from build123d import *

# Parameters (mm, degrees)
SKETCH2_W                       = 110
SKETCH2_H                       = 110
BOSS_EXTRUDE1_DEPTH             = 5.5
BOSS_EXTRUDE2_DEPTH             = 14
CUT_EXTRUDE5_REACH              = 110.823
SKETCH9_R                       = 1.3
CUT_EXTRUDE6_DEPTH              = 7.5
CUT_EXTRUDE9_REACH              = 109.547
SKETCH11_R                      = 9
BOSS_EXTRUDE7_DEPTH             = 9
BOSS_EXTRUDE7_DIRECTION_2_REACH = 119.904
BOSS_EXTRUDE10_DEPTH            = 9
CUT_EXTRUDE10_DEPTH             = 3.5
F_4_0_4_DIAMETER_HOLE3_D        = 4
FILLET1_R                       = 27.5
FILLET2_R                       = 40


with BuildPart() as part:
    # Sketch2 → Boss-Extrude1 (new body)
    with BuildSketch(Plane(origin=(0, 0, 0), x_dir=(1, 0, 0), z_dir=(0, 1, 0))):
        with Locations((-8.65, 8.65)):
            Rectangle(SKETCH2_W, SKETCH2_H)
    extrude(amount=BOSS_EXTRUDE1_DEPTH)

    # Sketch7 → Boss-Extrude2 (add)
    with BuildSketch(Plane(origin=(-8.65, 0, -8.65), x_dir=(-0.7071067811865479, 0, 0.7071067811865471), z_dir=(-0.7071067811865471, 0, -0.7071067811865479))):
        with BuildLine():
            Line((39.760240188, 5.5), (39.760240188, 15.95953406))
            ThreePointArc((39.760240188, 15.95953406), (42.812638822, 25.987954346), (50.934597235, 32.615181699))
            ThreePointArc((50.934597235, 32.615181699), (60.680796502, 64.420514285), (27.578950135, 67.712223286))
            Line((27.578950135, 67.712223286), (-10.597023433, 29.536249718))
            ThreePointArc((-10.597023433, 29.536249718), (-16.016342216, 21.425665997), (-17.919353903, 11.858580188))
            Line((-17.919353903, 11.858580188), (-17.919353903, 5.5))
            Line((-17.919353903, 5.5), (39.760240188, 5.5))
        make_face()
    extrude(amount=-BOSS_EXTRUDE2_DEPTH)

    # Sketch8 → Cut-Extrude5 (cut, up to next)
    with BuildSketch(Plane(origin=(-7.235786438, 0, -7.235786438), x_dir=(-0.7071067811865479, 0, 0.7071067811865471), z_dir=(-0.7071067811865471, 0, -0.7071067811865479)), mode=Mode.PRIVATE) as cut_extrude5_sk1:
        Polygon((13.613591207, 38.190515171), (42.604969235, 67.1818932), (57.45421164, 52.332650795), (28.462833611, 23.341272767), align=None)
    cut_extrude5_tool1 = extrude(cut_extrude5_sk1.sketch, amount=-CUT_EXTRUDE5_REACH, mode=Mode.PRIVATE) & part.part
    add(cut_extrude5_tool1.solids().sort_by_distance((-32.362049, 45.261583, 17.890476))[0], mode=Mode.SUBTRACT)

    # Sketch9 → Cut-Extrude6 (cut)
    with BuildSketch(Plane(origin=(1.249494937, 0, 1.249494937), x_dir=(0.7071067811865479, 0, -0.7071067811865471), z_dir=(0.7071067811865471, 0, 0.7071067811865479))):
        with Locations((-48.968930266, 65.767679638)):
            Circle(SKETCH9_R)
        with Locations((-56.039998078, 58.696611826)):
            Circle(SKETCH9_R)
        with Locations((-22.098872581, 24.755486329)):
            Circle(SKETCH9_R)
        with Locations((-15.027804769, 31.826554141)):
            Circle(SKETCH9_R)
    extrude(amount=-CUT_EXTRUDE6_DEPTH, mode=Mode.SUBTRACT)

    # Sketch11 → Cut-Extrude9 (cut, up to next)
    with BuildSketch(Plane(origin=(-8.65, 0, -8.65), x_dir=(-0.7071067811865479, 0, 0.7071067811865471), z_dir=(-0.7071067811865471, 0, -0.7071067811865479)), mode=Mode.PRIVATE) as cut_extrude9_sk1:
        with Locations((42.781745931, 52.50942749)):
            Circle(SKETCH11_R)
    cut_extrude9_tool1 = extrude(cut_extrude9_sk1.sketch, amount=-CUT_EXTRUDE9_REACH, mode=Mode.PRIVATE) & part.part
    add(cut_extrude9_tool1.solids().sort_by_distance((-38.901263, 52.509427, 21.601263))[0], mode=Mode.SUBTRACT)

    # Sketch17 → Boss-Extrude7 (add)
    with BuildSketch(Plane(origin=(1.249494937, 0, 1.249494937), x_dir=(0.7071067811865479, 0, -0.7071067811865471), z_dir=(0.7071067811865471, 0, 0.7071067811865479))):
        with BuildLine():
            Line((11.538994713, 28.541175194), (-25.457629791, 69.83354363))
            ThreePointArc((-25.457629791, 69.83354363), (-63.178338442, 66.082526396), (-52.072204394, 29.839240426))
            ThreePointArc((-52.072204394, 29.839240426), (-45.303905717, 24.316550965), (-42.760240188, 15.95953406))
            Line((-42.760240188, 15.95953406), (-42.760240188, 5.5))
            Line((-42.760240188, 5.5), (-39.760240188, 5.5))
            Line((-39.760240188, 5.5), (-39.760240188, 15.95953406))
            ThreePointArc((-39.760240188, 15.95953406), (-42.812638822, 25.987954346), (-50.934597235, 32.615181699))
            ThreePointArc((-50.934597235, 32.615181699), (-60.680796502, 64.420514285), (-27.578950135, 67.712223286))
            Line((-27.578950135, 67.712223286), (9.30583444, 26.537928118))
            ThreePointArc((9.30583444, 26.537928118), (13.46810778, 19.716615191), (14.919353903, 11.858580188))
            Line((14.919353903, 11.858580188), (14.919353903, 5.5))
            Line((14.919353903, 5.5), (17.919353903, 5.5))
            Line((17.919353903, 5.5), (17.919353903, 11.858580188))
            ThreePointArc((17.919353903, 11.858580188), (16.26984662, 20.78911712), (11.538994713, 28.541175194))
        make_face()
    extrude(amount=BOSS_EXTRUDE7_DEPTH)

    # Boss-Extrude7 direction 2: up to this face of the body (flat: up to its plane)
    boss_extrude7_direction_2_end = Plane(part.part.faces().sort_by_distance((-25.67440007, 34.90069961, 8.37440007))[0])
    # Sketch17 → Boss-Extrude7 direction 2 (add, up to the picked face)
    with BuildSketch(Plane(origin=(1.249494937, 0, 1.249494937), x_dir=(0.7071067811865479, 0, -0.7071067811865471), z_dir=(0.7071067811865471, 0, 0.7071067811865479)), mode=Mode.PRIVATE) as boss_extrude7_direction_2_sk1:
        with BuildLine():
            Line((11.538994713, 28.541175194), (-25.457629791, 69.83354363))
            ThreePointArc((-25.457629791, 69.83354363), (-63.178338442, 66.082526396), (-52.072204394, 29.839240426))
            ThreePointArc((-52.072204394, 29.839240426), (-45.303905717, 24.316550965), (-42.760240188, 15.95953406))
            Line((-42.760240188, 15.95953406), (-42.760240188, 5.5))
            Line((-42.760240188, 5.5), (-39.760240188, 5.5))
            Line((-39.760240188, 5.5), (-39.760240188, 15.95953406))
            ThreePointArc((-39.760240188, 15.95953406), (-42.812638822, 25.987954346), (-50.934597235, 32.615181699))
            ThreePointArc((-50.934597235, 32.615181699), (-60.680796502, 64.420514285), (-27.578950135, 67.712223286))
            Line((-27.578950135, 67.712223286), (9.30583444, 26.537928118))
            ThreePointArc((9.30583444, 26.537928118), (13.46810778, 19.716615191), (14.919353903, 11.858580188))
            Line((14.919353903, 11.858580188), (14.919353903, 5.5))
            Line((14.919353903, 5.5), (17.919353903, 5.5))
            Line((17.919353903, 5.5), (17.919353903, 11.858580188))
            ThreePointArc((17.919353903, 11.858580188), (16.26984662, 20.78911712), (11.538994713, 28.541175194))
        make_face()
    boss_extrude7_direction_2_tool1 = split(extrude(boss_extrude7_direction_2_sk1.sketch, amount=-BOSS_EXTRUDE7_DIRECTION_2_REACH, mode=Mode.PRIVATE), bisect_by=boss_extrude7_direction_2_end, keep=Keep.BOTH, mode=Mode.PRIVATE)
    add(boss_extrude7_direction_2_tool1.solids().sort_by(Axis((-4.257288, 48.445096, 6.756277), (-0.7071067811865471, 0, -0.7071067811865479)))[0])

    # Sketch25 → Boss-Extrude10 (add)
    with BuildSketch(Plane(origin=(1.249494937, 0, 1.249494937), x_dir=(0.7071067811865479, 0, -0.7071067811865471), z_dir=(0.7071067811865471, 0, 0.7071067811865479))):
        with BuildLine():
            ThreePointArc((-50.934597235, 32.615181699), (-42.812638822, 25.987954346), (-39.760240188, 15.95953406))
            Line((-39.760240188, 15.95953406), (-39.760240188, 5.5))
            Line((-39.760240188, 5.5), (-31.760240188, 5.5))
            add(Edge.make_bspline(
                [(-50.934597235, 32.615181699), (-42.286107378, 29.070948228), (-3.49892217, 18.530427319), (-31.760240188, 5.5)],
                knots=[0, 0, 0, 0, 1, 1, 1, 1], degree=3))
        make_face()
        with BuildLine():
            add(Edge.make_bspline(
                [(-5.279129206, 42.819047964), (9.40428973, 26.428022984), (8.919353903, 5.5)],
                knots=[0, 0, 0, 1, 1, 1], degree=2))
            Line((8.919353903, 5.5), (14.919353903, 5.5))
            Line((14.919353903, 5.5), (14.919353903, 11.858580188))
            ThreePointArc((14.919353903, 11.858580188), (13.46810778, 19.716615191), (9.30583444, 26.537928118))
            Line((9.30583444, 26.537928118), (-5.279129206, 42.819047964))
        make_face()
    extrude(amount=BOSS_EXTRUDE10_DEPTH)

    # Sketch26 → Cut-Extrude10 (cut)
    with BuildSketch(Plane.XZ):
        with BuildLine():
            Line((-2.35, -23.65), (-2.35, -63.65))
            Line((-2.35, -63.65), (46.35, -63.65))
            Line((46.35, -63.65), (46.35, 2.35))
            Line((46.35, 2.35), (23.65, 2.35))
            ThreePointArc((23.65, 2.35), (5.265223689, -5.265223689), (-2.35, -23.65))
        make_face()
    extrude(amount=-CUT_EXTRUDE10_DEPTH, mode=Mode.SUBTRACT)

    # Ø4.0 (4) Diameter Hole3 (through all)
    with Locations(Plane(origin=(0, 5.5, 0), x_dir=(1, 0, 0), z_dir=(0, 1, 0))):
        with Locations((38.35, -40.35), (38.35, -20.35), (38.35, -0.35)):
            f_4_0_4_diameter_hole3 = Hole(F_4_0_4_DIAMETER_HOLE3_D / 2)

    # Mirror1: Ø4.0 (4) Diameter Hole3 across plane
    add(f_4_0_4_diameter_hole3.mirror(Plane(origin=(-8.65, 0, -8.65), x_dir=(-0.7071067811865481, 0, 0.707106781186547), z_dir=(-0.7071067811865472, 0, -0.707106781186548))), mode=Mode.SUBTRACT)

    # Fillet1
    fillet1_edges = [part.edges().sort_by_distance(p)[0] for p in [
        (46.35, 4.5, -63.65),
    ]]
    fillet(fillet1_edges, radius=FILLET1_R)

    # Fillet2
    fillet2_edges = [part.edges().sort_by_distance(p)[0] for p in [
        (-63.65, 2.75, 46.35),
    ]]
    fillet(fillet2_edges, radius=FILLET2_R)


solid = part.part
Build history of the part. All positions in model axes, mm. A direction names the side the tool comes from. Give positions to 0.01 mm unless a question says otherwise; leave off trailing zeros. Loops run counter-clockwise (first coordinate to the right, second up) from the corner with the lowest first, then second, coordinate; pieces in that order, holes last. Notation, with made-up numbers: (41, -12) -> (86, -12) arc R16 cw to (86, 8) -> close; hole circle Ø6 at (33, -12.5). An arc over 180 degrees is marked (long way). Answer in a Markdown table with one row per item.
Item 1: Slice it at B-B on y = 50. Write the cut outline in (x, z), plus the area to 3 significant figures.
Findings below:
| item | result |
|---|---|
| outline | (-56.13, 38.83) -> (-45.01, 27.71) -> (-43.6, 29.13) -> (-46.21, 31.74) -> (-37.73, 40.23) -> (-44.1, 46.6) -> (-37.74, 52.96) -> (-39.87, 55.1) -> close; (-32.79, 15.49) -> (-14.09, -3.21) -> (2.18, 13.05) -> (-0.67, 15.9) -> (-7.03, 9.53) -> (-16.73, 19.23) -> (-25.21, 10.74) -> (-31.38, 16.9) -> close |
| area | 505 mm² |
Item 2: Slice it at A-A on z = -55.65. Write the cut outline in (x, y).
Findings below:
| item | result |
|---|---|
| outline | (-63.65, 0) -> (-59.65, 0) -> (-59.65, 5.5) -> (-63.65, 5.5) -> close; (-55.65, 0) -> (-39.65, 0) -> (-39.65, 5.5) -> (-55.65, 5.5) -> close; (-35.65, 0) -> (-19.65, 0) -> (-19.65, 5.5) -> (-35.65, 5.5) -> close; (-15.65, 0) -> (-2.35, 0) -> (-2.35, 3.5) -> (38.24, 3.5) -> (38.24, 5.5) -> (-15.65, 5.5) -> close |
Item 3: Tool access for faces 1 (the cylindrical face through (-52.244, 2.788, 34.322)), 2 (the flat face through (22, 3.5, -30)), 3 (the flat face through (-9.979, 20.234, 25.206)), 4 (the flat face through (-38.36, 59.86, 32.25)): list every direction of +Z, -Z, +X, -X, +Y, -Y with a clear straight run to the whole face (end or side of a thin tool).
Findings below:
| item | result |
|---|---|
| face 1 | +Z, -X, -Y |
| face 2 | -Z, +X, -Y |
| face 3 | +Z, +X, +Y |
| face 4 | none |
Item 4: Probe line 1 along Z through (x, y) = (38, 3); line 2 along Z through (x, y) = (38.35, 3.7); line 3 along Y through (x, z) = (26, -35.5). List the from-to ranges inside material, lowest first. Write a range as [from, to].
Findings below:
| item | result |
|---|---|
| line 1 | z = [2.35, 18.38], [22.32, 38.38], [42.32, 46.35] |
| line 2 | z = [-55.54, -1.65], [2.35, 18.35], [22.35, 38.35], [42.35, 46.35] |
| line 3 | y = [3.5, 5.5] |
Item 5: Slice it at C-C on x = 31.5. Write the cut outline in (y, z).
Findings below:
| item | result |
|---|---|
| outline | (0, 2.35) -> (3.5, 2.35) -> (3.5, -60.57) -> (5.5, -60.57) -> (5.5, 46.35) -> (0, 46.35) -> close |
Item 6: Flat gauge pins, fed straight in: P1, Ø2.5, axis at x = 38.35, z = 40.35, coming from the -Y side; P2, Ø1.5, axis at x = -48, y = 44.5, coming from the -Z side; P3, Ø1, axis at x = 33, y = 2, coming from the -Z side; P4, Ø8, axis at x = 31, z = -4, coming from the +Y side. Where does each tip first touch, or does it go through?
Findings below:
| item | result |
|---|---|
| P1 | passes through |
| P2 | stops at z = 29.95 |
| P3 | stops at z = 2.35 |
| P4 | stops at y = 5.5 |
Item 7: Mould opens along Z. For faces 5 (the cylindrical face through (40.348, 4.486, 0.262)), 6 (the flat face through (-22, 0, -9)), 7 (the flat face through (12.04, 8.63, -13.3)), 8 (the flat face through (-12, 32.6, 14.5)) say: pulls with the +Z half, pulls with the -Z half, needs draft (parallel to the pull), parting line crosses it, or undercut.
Findings below:
| item | result |
|---|---|
| face 5 | undercut |
| face 6 | needs draft |
| face 7 | pulls with the -Z half |
| face 8 | undercut |
